Autodesk Inventor part; units mm, degrees
ref_plane "YZ Plane" through (0, 0, 0) normal (1, 0, 0) x (0, 1, 0)
ref_plane "XZ Plane" through (0, 0, 0) normal (0, 1, 0) x (-1, 0, 0)
ref_plane "XY Plane" through (0, 0, 0) normal (0, 0, 1) x (1, 0, 0)
sketch "Sketch1" plane through (0, 0, 0) normal (1, 0, 0) x (0, 1, 0)
  line L0 (-7.5, -12.5) -> (7.5, -12.5)
  line L1 (7.5, -12.5) -> (7.5, 12.5)
  line L2 (7.5, 12.5) -> (-7.5, 12.5)
  line L3 (-7.5, 12.5) -> (-7.5, -12.5)
  line L4 (-7.5, -12.5) -> (7.5, 12.5) construction
  line L5 (7.5, -12.5) -> (-7.5, 12.5) construction
  point P0 (0, 0)
  dimension "d0" = 25
  dimension "d1" = 15
extrude "Extrusion1" add sketch "Sketch1" along normal blind 10
sketch "Sketch2" plane through (10, 0, 0) normal (1, 0, 0) x (0, 0, -1)
  line L0 (9.5, -4.5) -> (5.3472, -4.5)
  line L1 (9.5, -7.5) -> (9.5, -4.5)
  line L2 (9.5, -7.5) -> (22, -7.5)
  line L3 (22, 12.5) -> (22, -7.5)
  line L4 (-35, 12.5) -> (22, 12.5)
  line L5 (-35, 12.5) -> (-35, 59.5)
  line L6 (-45, 59.5) -> (-35, 59.5)
  line L7 (-45, 59.5) -> (-45, -7.5)
  line L8 (-45, -7.5) -> (-9.5, -7.5)
  line L9 (-9.5, -4.5) -> (-9.5, -7.5)
  line L10 (-5.3472, -4.5) -> (-9.5, -4.5)
  line L11 (-9.1, 2) -> (-5.3472, -4.5)
  line L12 (9.1, 2) -> (-9.1, 2)
  line L13 (5.3472, -4.5) -> (9.1, 2)
  line L14 (-9.5, -7.5) -> (9.5, -7.5)
  line L15 (-9.75, -7.25) -> (-44.75, -7.25)
  line L16 (-44.75, -7.25) -> (-44.75, 59.25)
  line L17 (-44.75, 59.25) -> (-35.25, 59.25)
  line L18 (-35.25, 59.25) -> (-35.25, 12.25)
  line L19 (-35.25, 12.25) -> (21.75, 12.25)
  line L20 (21.75, 12.25) -> (21.75, -7.25)
  line L21 (21.75, -7.25) -> (9.75, -7.25)
  line L22 (9.75, -7.25) -> (9.75, -4.25)
  line L23 (9.75, -4.25) -> (5.7802, -4.25)
  line L24 (5.7802, -4.25) -> (9.533, 2.25)
  line L25 (9.533, 2.25) -> (-9.533, 2.25)
  line L26 (-9.533, 2.25) -> (-5.7802, -4.25)
  line L27 (-5.7802, -4.25) -> (-9.75, -4.25)
  line L28 (-9.75, -4.25) -> (-9.75, -7.25)
  line L29 (-9.75, -7.25) -> (-9.75, -7.5)
  line L30 (-12.5, -7.5) -> (12.5, -7.5)
  line L31 (9.75, -7.25) -> (9.75, -7.5)
  line L32 (-12.5, -7.5) -> (12.5, -7.5)
  point P0 (0, 0)
  dimension "d4" = 0.25
extrude "Extrusion2" cut sketch "Sketch2" against normal blind 10 contours L1 L14 L9 L10 L11 L12 L13 L0 | L0 L13 L12 L11 L10 L9 L8 L29 L28 L27 L26 L25 L24 L23 L22 L31 L2 L1
properties part number "tester"
CAD build for the part. Positions are in the model's coordinates, mm. A direction names the side the tool comes from. Give positions to 0.01 mm unless a question says otherwise; leave off trailing zeros. Loops run counter-clockwise (first coordinate to the right, second up) from the corner with the lowest first, then second, coordinate; pieces in that order, holes last. Notation, with made-up numbers: M 41,48 L 61,48 A31 cw 61,77 Z; hole C -19.75,24.5 d9. An arc over 180 degrees is marked long. Answer in a Markdown table with one row per item. Add a question column.
Item 1: Band-saw the part on C-C on z = -7.5. Give the cut face in (x, y).
Item 2: Probe probe 1 along Y at (x, z) = (6.5, 5.5); probe 2 along Z at (x, y) = (1.5, -6); probe 3 along Z at (x, y) = (5, -0.75). List the from-to ranges inside material, lowest first.
Item 3: Tool access for faces 1 (the face through (10, 3, 0)), 2 (the face through (5, -4.25, -8)), 3 (the face through (5.07, -0.955, 7.683)): list every direction of +Z, -Z, +X, -X, +Y, -Y with a clear straight run to the whole face (end or side of a thin tool).
Item 4: Mould opens along Z. For faces 4 (the face through (5.07, -1.05, -7.63)), 5 (the face through (0, 3, 0)), 6 (the face through (5, 0, -12.5)) say: +Z half, -Z half, draft (parallel to the pull), parting line (faces both ways), or undercut.
Item 5: Band-saw the part on A-A on y = -6.5. Give the cut face in (x, z), then the cut area to 3 significant figures.
Item 6: Drop a flat-ended pin along its axis: P1, Ø4, axis at x = 4.5, z = -6.5, coming from the -Y side. Give the stop position or say it passes through.
Item 7: Band-saw the part on D-D on z = 0.25. Give the cut face in (x, y), then the cut area to 3 significant figures.
Item 8: Band-saw the part on B-B on x = 9.25. Give the cut face in (y, z), then the cut area to 3 significant figures.
Reply:
| question | item | result |
|---|---|---|
| 1 | outline | M 0,-4.25 L 10,-4.25 L 10,-1.27 L 0,-1.27 Z; M 0,2.25 L 10,2.25 L 10,7.5 L 0,7.5 Z |
| 2 | probe 1 | y = 2.25 to 7.5 |
| 2 | probe 2 | z = -12.5 to -9.75, 9.75 to 12.5 |
| 2 | probe 3 | z = -12.5 to -7.8, 7.8 to 12.5 |
| 3 | face 1 | +Z, -Z, +X, +Y, -Y |
| 3 | face 2 | +X, -X, -Y |
| 3 | face 3 | +X, -X |
| 4 | face 4 | undercut |
| 4 | face 5 | draft |
| 4 | face 6 | -Z half |
| 5 | outline | M 0,-12.5 L 10,-12.5 L 10,-9.75 L 0,-9.75 Z; M 0,9.75 L 10,9.75 L 10,12.5 L 0,12.5 Z |
| 5 | area | 55.0 mm^2 |
| 6 | P1 | stops at y = -4.25 |
| 7 | outline | M 0,2.25 L 10,2.25 L 10,7.5 L 0,7.5 Z |
| 7 | area | 52.5 mm^2 |
| 8 | outline | M -7.5,-12.5 L 7.5,-12.5 L 7.5,12.5 L -7.5,12.5 L -7.5,9.75 L -4.25,9.75 L -4.25,5.78 L 2.25,9.53 L 2.25,-9.53 L -4.25,-5.78 L -4.25,-9.75 L -7.5,-9.75 Z |
| 8 | area | 212 mm^2 |
